Part print with two shaded views. Sizes in mm from the minimum x, y, z corner. A direction names the side the tool comes from. Give positions to 0.01 mm unless a question says otherwise; leave off trailing zeros. Write each loop counter-clockwise with the first axis right and the second up, starting at its lowest first coordinate (ties: lowest second). Pieces come first, ordered by that corner, then holes.
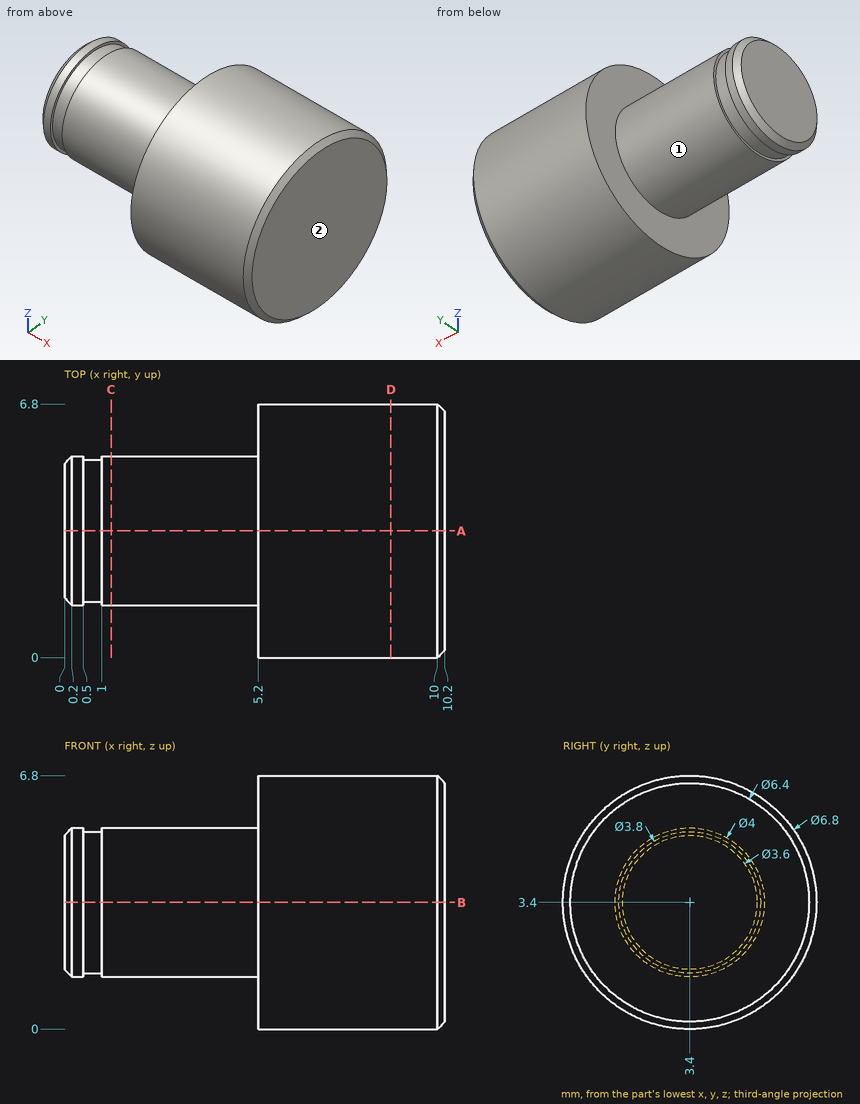
1) Saw through at A-A, the plane y = 3.4. Write the cut outline in (x, z), then the cut area to 3 significant figures.
Answers follow:
outline: (0, 1.6) - (0.2, 1.4) - (0.5, 1.4) - (0.5, 1.5) - (1, 1.5) - (1, 1.4) - (5.2, 1.4) - (5.2, 0) - (10, 0) - (10.2, 0.2) - (10.2, 6.6) - (10, 6.8) - (5.2, 6.8) - (5.2, 5.4) - (1, 5.4) - (1, 5.3) - (0.5, 5.3) - (0.5, 5.4) - (0.2, 5.4) - (0, 5.2) - close
area: 54.6 mm2
2) Saw through at D-D, the plane x = 8.75. Write the cut outline in (y, z), then the cut area to 3 significant figures.
Answers follow:
outline: circle Ø6.8 at (3.4, 3.4)
area: 36.3 mm2
3) Wall check: L1, parallel to Z at x = 6.75, y = 3.5; L2, parallel to Y at x = 0.75, z = 3.5; L3, parallel to X at y = 1.5, z = 4.25. Give the ranges that are in metal, low to high.
Answers follow:
L1: z = 0 to 6.8
L2: y = 1.5 to 5.3
L3: x = 5.2 to 10.2
4) 3-axis set-ups, long thin cutter, end or side, ignore diameter. For the marked faces 1 and 2: which of +Z, -Z, +X, -X, +Y, -Y reach the whole face in a straight line?
Answers follow:
face 1: -X
face 2: +Z, -Z, +X, +Y, -Y
5) Saw through at C-C, the plane x = 1.25. Write the cut outline in (y, z), then the cut area to 3 significant figures.
Answers follow:
outline: circle Ø4 at (3.4, 3.4)
area: 12.6 mm2
